Autodesk Inventor part; units mm, degrees
ref_plane "YZ Plane" through (0, 0, 0) normal (1, 0, 0) x (0, 1, 0)
ref_plane "XZ Plane" through (0, 0, 0) normal (0, 1, 0) x (-1, 0, 0)
ref_plane "XY Plane" through (0, 0, 0) normal (0, 0, 1) x (1, 0, 0)
sketch "Sketch1" plane through (0, 0, 0) normal (0, 1, 0) x (-1, 0, 0)
  line L0 (0, 0) -> (125, 0)
  line L1 (125, 0) -> (125, 120)
  line L2 (125, 120) -> (0, 120)
  line L3 (0, 120) -> (0, 0)
  dimension "d0" = 125
  dimension "d1" = 120
extrude "Extrusion1" add sketch "Sketch1" along normal blind 1.75
sketch "Sketch2" plane through (0, 1.75, 0) normal (0, 1, 0) x (1, 0, 0)
  line L0 (0, 0) -> (-125, 0)
  line L1 (-125, 0) -> (-125, -120)
  line L2 (-125, -120) -> (0, -120)
  line L3 (0, -120) -> (0, 0)
  line L4 (-125, 0) -> (-119.2077, 0)
  line L5 (-125, -4.4946) -> (-125, 0)
  line L6 (-125, 0) -> (-123.25, 0)
  line L7 (-123.25, 0) -> (-123.25, -1.75)
  line L8 (-123.25, -1.75) -> (-125, -1.75)
  line L9 (-125, -1.75) -> (-125, 0)
  line L10 (0, -120) -> (-1.75, -120)
  line L11 (-1.75, -120) -> (-1.75, -118.25)
  line L12 (-1.75, -118.25) -> (0, -118.25)
  line L13 (0, -118.25) -> (0, -120)
  line L14 (-1.75, -118.25) -> (-123.25, -118.25)
  line L15 (-123.25, -118.25) -> (-123.25, -1.75)
  line L16 (-123.25, -1.75) -> (-1.75, -1.75)
  line L17 (-1.75, -1.75) -> (-1.75, -118.25)
  dimension "d4" = 1.75
  dimension "d5" = 1.75
  dimension "d6" = 1.75
  dimension "d7" = 1.75
extrude "Extrusion2" add sketch "Sketch2" along normal blind 65 contours L3 L12 L17 L16 L7 L0 | L3 L2 L11 L12 | L7 L8 L1 L0 | L11 L2 L1 L8 L15 L14
sketch "Sketch3" plane through (0, 0, 120) normal (1, 0, 0) x (0, 0, -1)
  line L0 (0, 0) -> (120, 0)
  line L1 (120, 0) -> (120, 66.75)
  line L2 (0, 66.75) -> (120, 66.75)
  line L3 (0, 0) -> (0, 66.75)
sketch "Sketch4" plane through (0, 0, 0) normal (0, 0, -1) x (-1, 0, 0)
  line L0 (0, 0) -> (1.75, 0)
  line L1 (1.75, 0) -> (1.75, 30)
  line L2 (1.75, 30) -> (0, 30)
  line L3 (0, 30) -> (0, 0)
  line L4 (1.75, 30) -> (16.75, 30)
  line L5 (16.75, 30) -> (16.75, 0)
  line L6 (16.75, 0) -> (1.75, 0)
  line L7 (1.75, 0) -> (1.75, 30)
  line L8 (0, 0) -> (55, 0)
  line L9 (55, 0) -> (55, 1.75)
  line L10 (55, 1.75) -> (0, 1.75)
  line L11 (0, 1.75) -> (0, 0)
  line L12 (16.75, 1.75) -> (46.75, 1.75)
  line L13 (46.75, 1.75) -> (46.75, 30)
  line L14 (46.75, 30) -> (16.75, 30)
  line L15 (16.75, 30) -> (16.75, 1.75)
  dimension "d10" = 1.75
  dimension "d11" = 30
  dimension "d12" = 15
  dimension "d13" = 30
  dimension "d14" = 55
  dimension "d15" = 1.75
  dimension "d16" = 30
extrude "Extrusion3" cut sketch "Sketch4" against normal blind 4 contours L5 L14 L13 L10
sketch "Sketch5" plane through (-125, 0, 120) normal (0, 0, 1) x (1, 0, 0)
  line L0 (125, 0) -> (125, 66.75)
  line L1 (0, 66.75) -> (125, 66.75)
  line L2 (0, 0) -> (125, 0)
  line L3 (125, 0) -> (125, 1.75)
  line L4 (125, 1.75) -> (0, 1.75)
  line L5 (0, 1.75) -> (0, 0)
  line L6 (125, 1.75) -> (123.25, 1.75)
  line L7 (123.25, 1.75) -> (123.25, 66.75)
  line L8 (123.25, 66.75) -> (125, 66.75)
  line L9 (125, 66.75) -> (125, 1.75)
  line L10 (123.25, 1.75) -> (73.25, 1.75)
  line L11 (73.25, 1.75) -> (73.25, 31.75)
  line L12 (73.25, 31.75) -> (123.25, 31.75)
  line L13 (123.25, 31.75) -> (123.25, 1.75)
  dimension "d19" = 1.75
  dimension "d20" = 1.75
  dimension "d21" = 50
  dimension "d22" = 30
extrude "Extrusion4" cut sketch "Sketch5" against normal blind 8621077.25 contours L4 L11 L12 L7
properties part number "Case"
Verification items for the finished model (mm, model axes). A direction names the side the tool comes from. Round coordinates to 2 decimals unless told otherwise and drop trailing zeros. Order: outer loops, then holes, each group sorted by start corner. A loop starts at its lowest first (then second) coordinate and runs counter-clockwise, first axis right, second up. Notation, with made-up numbers: (-28.75, 44.5) - (25.25, 44.5) arc R29 cw to (25.25, 82.5) - close; hole circle Ø8 at (-25, 85.5). An arc over 180 degrees is marked (long way). Use CSV: the item, a comma, the result in double quotes. Start each with the question number.
1) Section check C-C, the plane y = 12. Record the cut outline in (x, z).
2) Thickness scan on L1, parallel to X at y = 12, z = 54.5; L2, parallel to Z at x = -47, y = 36; L3, parallel to Y at x = -61, z = 62. Record the ranges inside material, lowest first.
3) Section check D-D, the plane x = -107.5. Record the cut outline in (y, z), plus the area to 4 significant figures.
4) Section check A-A, the plane x = -21. Record the cut outline in (y, z).
5) Go/stop test with a flat-tipped pin: P1, Ø0.9, axis at y = 23.5, z = 1, coming from the +X side. Record where the tip stops, or that it passes through.
6) Access from +Z, -Z, +X, -X, +Y, -Y to the whole of each face (thin tool, end or side, straight path). Record for faces 4 (the flat face through (-125, 33, 59)), 5 (the flat face through (-123.25, 34, 61)).
7) Section check B-B, the plane y = 50. Record the cut outline in (x, z), plus the area to 3 significant figures.
8) Mould release check, pull along Z, two halves, no side actions. Record for faces 1 (the flat face through (-77, 40, 120)), 2 (the flat face through (-77, 41, 1.75)), 3 (the flat face through (-76, 40, 0)): +Z half, -Z half, draft (parallel to the pull), parting line (faces both ways), or undercut.
Answers:
1,outline,"(-125, 0) - (-51.75, 0) - (-51.75, 1.75) - (-123.25, 1.75) - (-123.25, 118.25) - (-51.75, 118.25) - (-51.75, 120) - (-125, 120) - close; (-1.75, 0) - (0, 0) - (0, 120) - (-1.75, 120) - close"
2,L1,"x = -125 to -123.25, -1.75 to 0"
2,L2,"z = 0 to 1.75, 118.25 to 120"
2,L3,"y = 0 to 1.75"
3,outline,"(0, 0) - (66.75, 0) - (66.75, 1.75) - (1.75, 1.75) - (1.75, 118.25) - (66.75, 118.25) - (66.75, 120) - (0, 120) - close"
3,area,"437.5 mm²"
4,outline,"(0, 0) - (1.75, 0) - (1.75, 120) - (0, 120) - close; (31.75, 0) - (66.75, 0) - (66.75, 1.75) - (31.75, 1.75) - close; (31.75, 118.25) - (66.75, 118.25) - (66.75, 120) - (31.75, 120) - close"
5,P1,"stops at x = 0"
6,face 4,"+Z, -Z, -X, +Y, -Y"
6,face 5,"+Y"
7,outline,"(-125, 0) - (0, 0) - (0, 120) - (-125, 120) - close; hole (-123.25, 1.75) - (-1.75, 1.75) - (-1.75, 118.25) - (-123.25, 118.25) - close"
7,area,"845 mm²"
8,face 1,"+Z half"
8,face 2,"undercut"
8,face 3,"-Z half"
